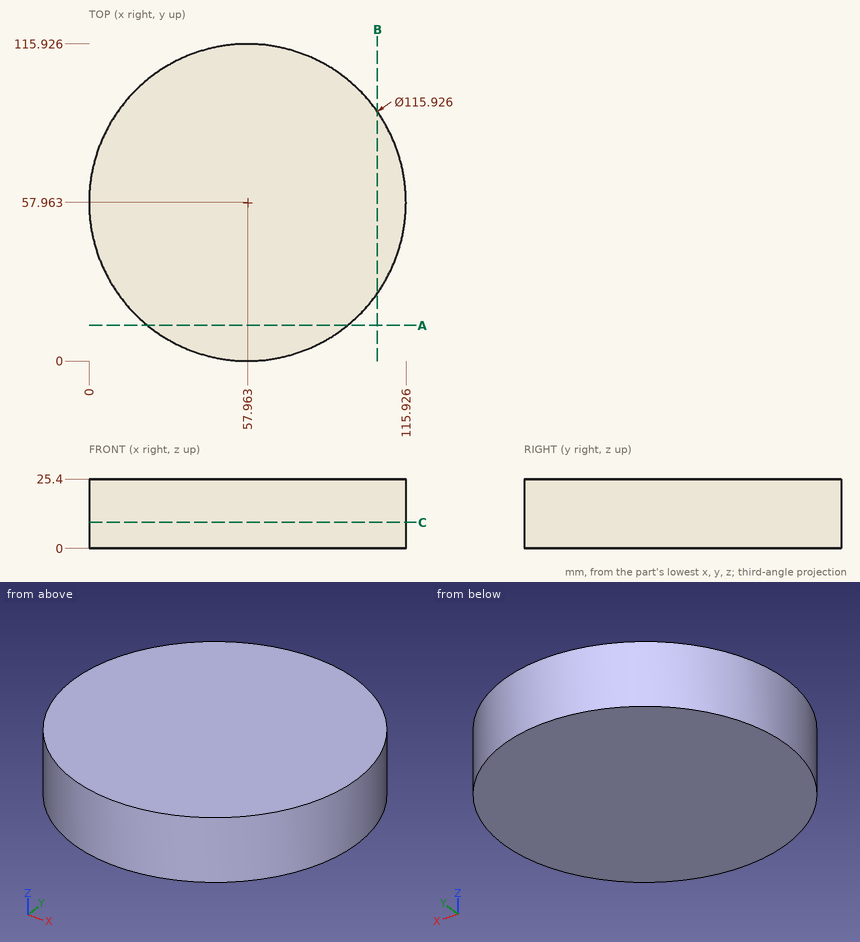
Could you check a few things on this drawing? It's one solid part, dimensions in mm from its lowest x, y, z. Round coordinates to 2 decimals unless told otherwise and drop trailing zeros. Write each loop counter-clockwise with the first axis right and the second up, starting at its lowest first coordinate (ties: lowest second). Pieces come first, ordered by that corner, then holes. Notation, with made-up numbers: (-37, 62.25) -> (-10, 62.25) arc R10 cw to (-10, 76.25) -> close; hole circle Ø6 at (65.25, -20.75). An arc over 180 degrees is marked (long way). One line per question, with ' | ' between items. Start each with the question number.
1) Suppose I cut it at C-C on z = 9.5. Write out the boundary of the cut face in (x, y) (1 decimal), then the cut area to 3 significant figures.
2) I'm going to push flat-ended pins straight in: P1, Ø2, axis at x = 84.5, z = 3, coming from the +Y side; P2, Ø8, axis at x = 51, z = 8, coming from the +Y side; P3, Ø1, axis at x = 37, z = 20, coming from the +Y side. Where does each tip first touch, or does it pass through?
3) Suppose I cut it at B-B on x = 105.5. Write out the boundary of the cut face in (y, z).
4) Suppose I cut it at A-A on y = 13. Write out the boundary of the cut face in (x, z).
5) I need wall thicknesses on line 1 (X direction, y = 59, z = 15.25); line 2 (X direction, y = 106.5, z = 14.25) (1 decimal); line 3 (Y direction, x = 72, z = 18.5) (1 decimal). Which ranges of each line are inside material? Lowest first, please. Write a range as [from, to].
Return value:
1) outline: circle Ø115.9 at (58, 58) | area: 10,600 mm2
2) P1: stops at y = 110 | P2: stops at y = 115.85 | P3: stops at y = 112.19
3) outline: (24.8, 0) -> (91.13, 0) -> (91.13, 25.4) -> (24.8, 25.4) -> close
4) outline: (21.38, 0) -> (94.54, 0) -> (94.54, 25.4) -> (21.38, 25.4) -> close
5) line 1: x = [0.01, 115.92] | line 2: x = [26.3, 89.6] | line 3: y = [1.7, 114.2]
